CAD build for the part. Positions are in the model's coordinates, mm. Round coordinates to 2 decimals unless told otherwise and drop trailing zeros. Loops run counter-clockwise (first coordinate to the right, second up) from the corner with the lowest first, then second, coordinate; pieces in that order, holes last. Notation, with made-up numbers: M -2,-24 L 45,-24 A26 ccw 45,10 Z; hole C 36.25,60.25 d1. An arc over 180 degrees is marked long. Put each result on its own line as item: value. Start each with the question number.
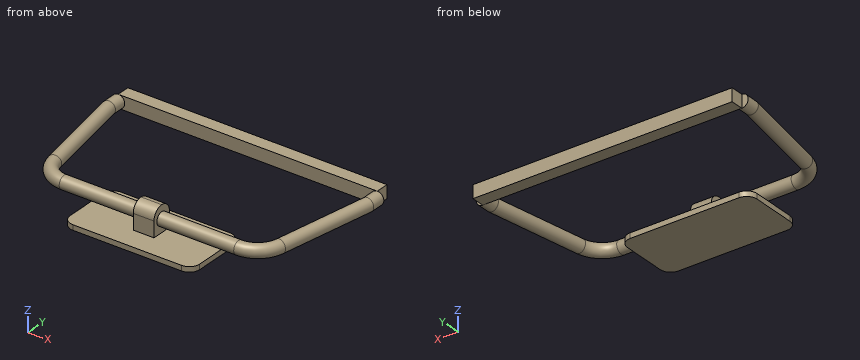
from build123d import *

# Parameters (mm, degrees)
F0_R          = 12.5
F4_DEPTH      = 25
F5_W          = 40
F5_H          = 40
F6_DEPTH      = 25
F6_DEPTH_BACK = 25
F7_R          = 19.99999
F9_DEPTH      = 10


# Not quite as in the source:
# - a fillet or chamfer is up to 0.001 mm smaller than in the source, because OpenCascade refuses the exact size


with BuildPart() as f2:
    # F2: sweep along a path in F1
    with BuildLine(Plane.XY) as f2_path:
        Line((-465.6524967789, 0), (-465.6524967789, -25))
        Line((-465.6524967789, -25), (-433.2643322113, -208.6824088833))
        ThreePointArc((-433.2643322113, -208.6824088833), (-416.163325045, -238.3022221559), (-384.0239445606, -250))
        Line((-384.0239445606, -250), (-47.2810489972, -250))
        ThreePointArc((-47.2810489972, -250), (-15.1416685129, -238.3022221559), (1.9593386534, -208.6824088833))
        Line((1.9593386534, -208.6824088833), (34.3475032211, -25))
        Line((34.3475032211, -25), (34.3475032211, 0))
    # F0 (on Front) → F2 (sweep)
    with BuildSketch(Plane.XZ):
        with Locations((-465.6524967789, 0)):
            Circle(F0_R)
    sweep(path=f2_path.line, transition=Transition.RIGHT)

    # F3 (on face) → F4 (join)
    with BuildSketch(Plane(origin=(0, 0, 0), x_dir=(-1, 0, 0), z_dir=(0, 1, 0))):
        with BuildLine():
            Line((465.6524967789, 12.5), (-34.3475032211, 12.5))
            Line((-34.3475032211, 12.5), (-34.3475032211, -12.5))
            Line((-34.3475032211, -12.5), (465.6524967789, -12.5))
            ThreePointArc((465.6524967789, -12.5), (453.1524967789, 0), (465.6524967789, 12.5))
        make_face()
        with BuildLine():
            Line((465.6524967789, -12.5), (465.6524967789, 12.5))
            ThreePointArc((465.6524967789, 12.5), (453.1524967789, 0), (465.6524967789, -12.5))
        make_face()
    extrude(amount=F4_DEPTH)

    # F5 (on Top) → F6 (join, two sides)
    with BuildSketch(Plane.XY) as f6_sk:
        with Locations((-215.5239445606, -250)):
            Rectangle(F5_W, F5_H)
    extrude(amount=F6_DEPTH)
    extrude(f6_sk.sketch, amount=-F6_DEPTH_BACK)

    # F7 (radius 20 in the source; OpenCascade refuses exactly that, so slightly less here)
    f7_edges = [f2.edges().sort_by_distance(p)[0] for p in [
        (-215.523945, -230, 25),
        (-215.523945, -270, 25),
    ]]
    fillet(f7_edges, radius=F7_R)

    # F8 (on face) → F9 (join)
    with BuildSketch(Plane(origin=(0, 0, -25), x_dir=(1, 0, 0), z_dir=(0, 0, -1))):
        with BuildLine():
            Line((-110.5239445606, 312.5), (-320.5239445606, 312.5))
            ThreePointArc((-320.5239445606, 312.5), (-334.6660801844, 306.6421356237), (-340.5239445606, 292.5))
            Line((-340.5239445606, 292.5), (-340.5239445606, 207.5))
            ThreePointArc((-340.5239445606, 207.5), (-334.6660801844, 193.3578643763), (-320.5239445606, 187.5))
            Line((-320.5239445606, 187.5), (-110.5239445606, 187.5))
            ThreePointArc((-110.5239445606, 187.5), (-96.3818089369, 193.3578643763), (-90.5239445606, 207.5))
            Line((-90.5239445606, 207.5), (-90.5239445606, 292.5))
            ThreePointArc((-90.5239445606, 292.5), (-96.3818089369, 306.6421356237), (-110.5239445606, 312.5))
        make_face()
    extrude(amount=F9_DEPTH)


solid = f2.part
(1) Drill centre lines: line 1 along Y through (x, z) = (-354, 1); line 2 along X through (y, z) = (-49, 11.5); line 3 along Y through (x, z) = (-126.5, -28.5). Where is each one in solid material? Low to high.
(2) Flat gauge pins, fed straight in: pin 1 Ø12 at (x, y) = (-161, -216) entering from +Z; pin 2 Ø20 at (x, z) = (-165, 3) entering from -Y; pin 3 Ø10 at (x, z) = (-471, -3.5) entering from +Y. Where does each tip first touch, or does it go through?
(3) Cut at A-A on x = -312.5. List the corners of the cut face in (y, z).
(4) Cut at B-B on x = -55.5. List the corners of the cut face in (y, z).
Taken from the geometry:
1. line 1: -262.46 to -237.54, 0 to 25
1. line 2: -466.4 to -456.45, 25.14 to 35.09
1. line 3: -312.5 to -187.5
2. pin 1: z = -25
2. pin 2: y = -262.5
2. pin 3: y = 0
3. outline: M -312.5,-35 L -187.5,-35 L -187.5,-25 L -312.5,-25 Z; C -250,0 d25; M 0,-12.5 L 25,-12.5 L 25,12.5 L 0,12.5 Z
4. outline: C -250,0 d25; M 0,-12.5 L 25,-12.5 L 25,12.5 L 0,12.5 Z
